Can you work these out from the model? Positions are in its coordinate system, mm. Give positions to 0.01 mm unless a question says otherwise; leave off trailing zeros. Write each loop counter-clockwise with the first axis right and the second up, starting at its lowest first coordinate (ties: lowest second). Pieces come first, ordered by that corner, then holes. Notation, with made-up numbers: (21, 59) -> (58, 59) arc R27 cw to (58, 89) -> close; hole circle Ø9 at (-25, 13). An arc over 180 degrees is marked (long way). One line per item, written item: value.
from build123d import *

# Parameters (mm, degrees)
F1_DEPTH = 1
F2_R     = 1
F2_R_2   = 0.5
F3_DEPTH = 1.001


with BuildPart() as f1:
    # F0 (on Front) → F1 (new body)
    with BuildSketch(Plane.XZ):
        Polygon((-3, 21), (-2, 0), (2, 0), (3, 21), align=None)
        with BuildLine():
            ThreePointArc((3, 21), (0, 24.146257), (-3, 21))
            Line((-3, 21), (3, 21))
        make_face()
        with BuildLine():
            Line((2, 0), (-2, 0))
            ThreePointArc((-2, 0), (0, -1.907028), (2, 0))
        make_face()
    extrude(amount=F1_DEPTH)

    # F2 (on face) → F3 (cut, through all)
    with BuildSketch(Plane.XZ.offset(1)):
        with Locations((0, 21.142857)):
            Circle(F2_R)
        Circle(F2_R_2)
    extrude(amount=-F3_DEPTH, mode=Mode.SUBTRACT)


solid = f1.part
1) Will these pins go through, and if not, where does the flat tip stop? pin 1 (2 mm diameter, centred on x = 1.5, z = 8, fed in from +Y); pin 2 (1.6 mm diameter, centred on x = 0, z = 21.14, fed in from +Y) (3 decimals).
Answer list:
pin 1: stops at y = 0
pin 2: passes through
2) I need wall thicknesses on L1, parallel to X at y = -0.5, z = 21.25; L2, parallel to Z at x = 0.75, y = -0.1; L3, parallel to X at y = -0.2, z = 5.25. Which ranges of each line are inside material? Lowest first, please.
Answer list:
L1: x = -3 to -0.99, 0.99 to 3
L2: z = -1.76 to 20.48, 21.8 to 24.05
L3: x = -2.25 to 2.25
3) If we section it at C-C (z = 18.25): Write out the boundary of the cut face in (x, y).
Answer list:
outline: (-2.87, -1) -> (2.87, -1) -> (2.87, 0) -> (-2.87, 0) -> close
4) If we section it at A-A (x = 0): Write out the boundary of the cut face in (y, z).
Answer list:
outline: (-1, -1.91) -> (0, -1.91) -> (0, -0.5) -> (-1, -0.5) -> close; (-1, 0.5) -> (0, 0.5) -> (0, 20.14) -> (-1, 20.14) -> close; (-1, 22.14) -> (0, 22.14) -> (0, 24.15) -> (-1, 24.15) -> close
5) If we section it at D-D (x = 1.75): Write out the boundary of the cut face in (y, z).
Answer list:
outline: (-1, -0.88) -> (0, -0.88) -> (0, 23.58) -> (-1, 23.58) -> close
6) If we section it at B-B (y = -0.2): Write out the boundary of the cut face in (x, z), and give its area (3 significant figures).
Answer list:
outline: (-3, 21) -> (-2, 0) arc R2 ccw to (2, 0) -> (3, 21) arc R3 ccw (long way) to start; hole circle Ø2 at (0, 21.14); hole circle Ø1 at (0, 0)
area: 122 mm^2
